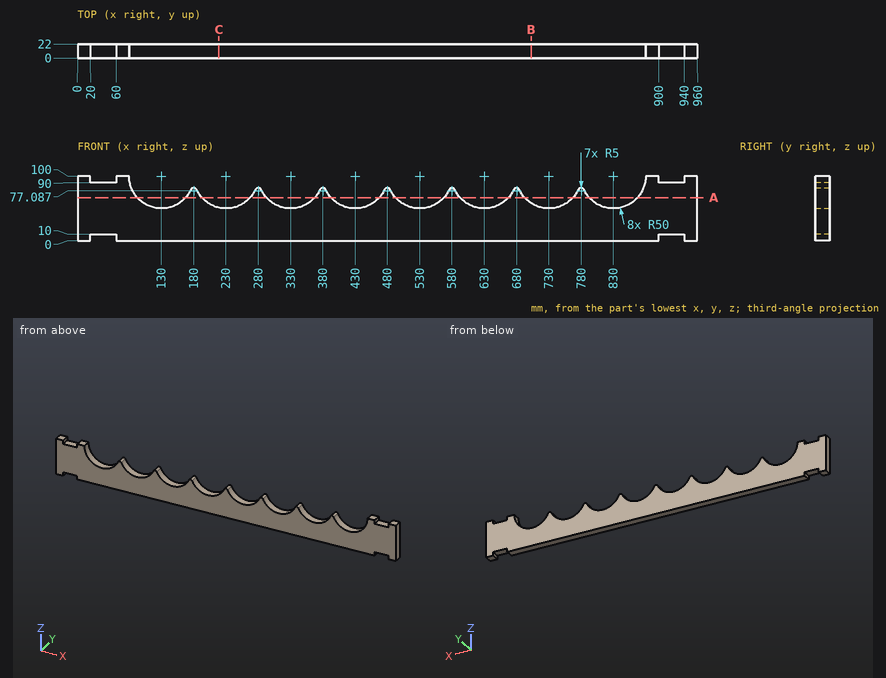
Input: dimensioned drawing with shaded views. Units: mm. Origin: part minimum x, y, z. Give positions to 0.01 mm unless a question says otherwise; leave off trailing zeros. Write each loop counter-clockwise with the first axis right and the second up, starting at its lowest first coordinate (ties: lowest second). Pieces come first, ordered by that corner, then holes.
1. Section query B-B (x = 702.5). Return the cut outline in (y, z).
2. Section query C-C (x = 219). Return the cut outline in (y, z) (3 decimals).
3. Section query A-A (z = 67). Count the separate pieces of the cut face and the enclosed holes in it, then the cut area to 3 significant figures.
4. First-contact query: pin 1 (11 mm diameter, centred on x = 41.5, y = 8.5, fed in from -Z); pin 2 (4 mm diameter, centred on x = 578.5, y = 4, fed in from +Z). Flat tips, straight axial feed; report the tip coordinate or a pass-through.
5. Material intervals for line 1 along Z through (x, y) = (42, 3.5); line 2 along Z through (x, y) = (320, 2); line 3 along X through (y, z) = (12.25, 82.5), sorted ascending.
Output values:
1. outline: (0, 0) - (22, 0) - (22, 58.24) - (0, 58.24) - close
2. outline: (0, 0) - (22, 0) - (22, 51.225) - (0, 51.225) - close
3. separate pieces: 9
3. enclosed holes: 0
3. area: 7,900 mm2
4. pin 1: stops at z = 10
4. pin 2: stops at z = 82.09
5. line 1: z = 10 to 90
5. line 2: z = 0 to 51.01
5. line 3: x = 0 to 83.16, 876.84 to 960
